from build123d import *

# Parameters (mm, degrees)
F0_R     = 32.773688
F1_DEPTH = 78.74
F2_R     = 25.62025
F3_DEPTH = 65.532
F4_R     = 5.08
F5_R     = 11.468996
F5_R_2   = 7.838538
F6_DEPTH = 42.672


with BuildPart() as f1:
    # F0 (on Top) → F1 (new body)
    with BuildSketch(Plane.XY):
        Circle(F0_R)
    extrude(amount=F1_DEPTH)

    # F2 (on Top) → F3 (cut)
    with BuildSketch(Plane.XY):
        Circle(F2_R)
    extrude(amount=F3_DEPTH, mode=Mode.SUBTRACT)

    # F4
    f4_edges = [f1.edges().sort_by_distance(p)[0] for p in [
        (-25.62025, 0, 0),
        (-25.62025, 0, 65.532),
    ]]
    fillet(f4_edges, radius=F4_R)

    # F5 (on Front) → F6 (join)
    with BuildSketch(Plane.XZ):
        with Locations((0, 29.404234)):
            Circle(F5_R)
        with Locations((0, 29.404234)):
            Circle(F5_R_2, mode=Mode.SUBTRACT)
    extrude(amount=-F6_DEPTH)


solid = f1.part
Can you work these out from the model? Positions are in its coordinate system, mm. A direction names the side the tool comes from. Give positions to 0.01 mm unless a question says otherwise; leave off trailing zeros. Write each loop counter-clockwise with the first axis right and the second up, starting at its lowest first coordinate (ties: lowest second). Pieces come first, ordered by that corner, then holes. Notation, with made-up numbers: M 1,59 L 9,59 A28 ccw 9,91 Z; hole C 81,6 d11. An arc over 180 degrees is marked long. Answer in a Markdown table with one row per item. Add a question column.
Item 1: For pin 1 Ø12 at (x, z) = (-20, 65) entering from -Y; pin 2 Ø3 at (x, z) = (-18, 17.5) entering from +Y; pin 3 Ø5 at (y, z) = (5, 58.5) entering from -X; pin 4 Ø18 at (x, z) = (0, 29.4) entering from +Y, each with a flat end and sliding along its axis, tell me the tip position at first contact or that it passes through.
Item 2: Imagine slicing it at D-D, the plane z = 69. Write out the boundary of the cut face in (x, y), plus the area to 3 significant figures.
Item 3: On a 3-axis mill with a long thin cutter (end or side, diameter ignored), from which of +Z, -Z, +X, -X, +Y, -Y can I reach the whole of each face in a straight line? I mean faces 1 (the flat face through (-3, 42.672, 22)), 2 (the flat face through (0, 0, 78.74)), 3 (the cylindrical face through (-7.83, 37.17, 29.75)), 4 (the cylindrical face through (-1.02, 12.64, 37.176)), 5 (the flat face through (-3, 0, 22)). Say none if no direction works.
Item 4: Imagine slicing it at B-B, the plane z = 42. Write out the boundary of the cut face in (x, y), plus the area to 3 significant figures.
Item 5: Imagine slicing it at A-A, the plane x = 0. Write out the boundary of the cut face in (y, z).
Item 6: Imagine slicing it at C-C, the plane y = 13.5. State how many separate pieces and enclosed holes the cut face has, plus the area to 3 significant figures.
Item 7: Please list where these lines run through material, in increasing order: L1, parallel to Z at x = 0, y = 36.75; L2, parallel to Y at x = 0, z = 47; L3, parallel to Z at x = -9.5, y = 7.5.
Item 8: We'd pull the mould along Z, two halves only. Please class faces 6 (the cylindrical face through (10.594, 36.603, 25.012)), 7 (the flat face through (-9.9, 29.3, 0)), 8 (the flat face through (0, 0, 65.532)): released by +Z, released by -Z, zero draft, split by the parting line, or undercut.
Evaluation:
| question | item | result |
|---|---|---|
| 1 | pin 1 | stops at y = -29.63 |
| 1 | pin 2 | stops at y = 28.32 |
| 1 | pin 3 | stops at x = -32.68 |
| 1 | pin 4 | stops at y = 42.67 |
| 2 | outline | C 0,0 d65.55 |
| 2 | area | 3,370 mm² |
| 3 | face 1 | +Z, -Z, +X, -X, +Y |
| 3 | face 2 | +Z, +X, -X, +Y, -Y |
| 3 | face 3 | +Y |
| 3 | face 4 | none |
| 3 | face 5 | -Z |
| 4 | outline | C 0,0 d65.55; hole C 0,0 d51.24 |
| 4 | area | 1,310 mm² |
| 5 | outline | M -32.77,0 L -30.7,0 A5.08 ccw -25.62,5.08 L -25.62,60.45 A5.08 cw -20.54,65.53 L 20.54,65.53 A5.08 cw 25.62,60.45 L 25.62,40.87 L 0,40.87 L 0,37.24 L 25.62,37.24 L 25.62,21.57 L 0,21.57 L 0,17.94 L 25.62,17.94 L 25.62,5.08 A5.08 ccw 30.7,0 L 32.77,0 L 32.77,17.94 L 42.67,17.94 L 42.67,21.57 L 32.77,21.57 L 32.77,37.24 L 42.67,37.24 L 42.67,40.87 L 32.77,40.87 L 32.77,78.74 L -32.77,78.74 Z |
| 6 | separate pieces | 2 |
| 6 | enclosed holes | 1 |
| 6 | area | 2,070 mm² |
| 7 | L1 | z = 17.94 to 21.57, 37.24 to 40.87 |
| 7 | L2 | y = -32.77 to -25.62, 25.62 to 32.77 |
| 7 | L3 | z = 22.98 to 35.83, 65.53 to 78.74 |
| 8 | face 6 | split by the parting line |
| 8 | face 7 | released by -Z |
| 8 | face 8 | undercut |
